Model file for the job. Use its own axes, mm. Give positions to 0.01 mm unless a question says otherwise; leave off trailing zeros. Order: outer loops, then holes, each group sorted by start corner. A loop starts at its lowest first (then second) coordinate and runs counter-clockwise, first axis right, second up. Notation, with made-up numbers: (56, -28.5) - (90, -28.5) arc R18 ccw to (90, -24.5) - close; hole circle Ø3 at (-38.75, -23). An arc over 180 degrees is marked (long way). Return JSON: item names as keys, results as strings. Group by question number.
from build123d import *

# Parameters (mm, degrees)
SKETCH_W      = 473.075
SKETCH_H      = 493.7252
SKETCH_R      = 34.925
EXTRUDE_DEPTH = 5.9944


with BuildPart() as part:
    # Sketch → Extrude (new body)
    with BuildSketch(Plane.XY.offset(762)):
        with Locations((236.5375, 246.8626)):
            Rectangle(SKETCH_W, SKETCH_H)
        with Locations((236.5502, 123.4186)):
            Circle(SKETCH_R, mode=Mode.SUBTRACT)
    extrude(amount=EXTRUDE_DEPTH)


solid = part.part
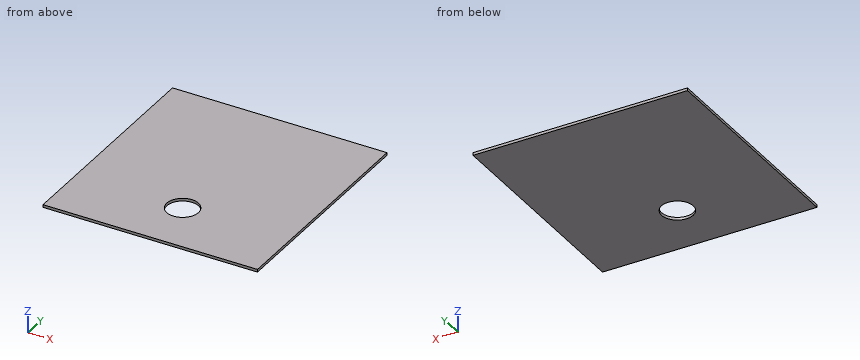
(1) Slice it at A-A (y = 140.5). Give the cut face in (x, z) (3 decimals).
(2) Drill centre lines: L1, parallel to X at y = 130, z = 766.1 (3 decimals); L2, parallel to X at y = 139, z = 763.1 (3 decimals). Where is each one in solid material? Low to high.
(3) Slice it at B-B (z = 764.7). Give the cut face in (x, y) (3 decimals), and give its area (3 significant figures).
Result set:
{
 "1": {"outline": "(0, 762) - (206.087, 762) - (206.087, 767.994) - (0, 767.994) - close; (267.013, 762) - (473.075, 762) - (473.075, 767.994) - (267.013, 767.994) - close"},
 "2": {"L1": "x = 0 to 202.251, 270.849 to 473.075", "L2": "x = 0 to 205.294, 267.807 to 473.075"},
 "3": {"outline": "(0, 0) - (473.075, 0) - (473.075, 493.725) - (0, 493.725) - close; hole circle Ø69.85 at (236.55, 123.419)", "area": "230,000 mm²"}
}
